from build123d import *

# Parameters (mm, degrees)
F0_W      = 78.632404
F0_H      = 78.044064
F1_DEPTH  = 19.05
F7_R      = 19.67966
F8_DEPTH  = 25.4
F9_R      = 25.337788
F10_DEPTH = 88.9
F11_W     = 78.605324
F11_H     = 78.906078
F12_DEPTH = 19.05
F13_R     = 19.066656
F14_DEPTH = 19.05
F6_R      = 6.832472
F15_DEPTH = 304.8
F4_R      = 6.169539
F16_DEPTH = 25.4
F3_R      = 6.600699
F17_DEPTH = 25.4
F5_R      = 6.490494
F18_DEPTH = 25.4
F19_R     = 6.482052
F19_R_2   = 6.426585
F19_R_3   = 6.219267
F19_R_4   = 6.38041
F20_DEPTH = 25.4


with BuildPart() as f1:
    # F0 (on Top) → F1 (new body)
    with BuildSketch(Plane.XY):
        with Locations((-12.092622, -33.094514)):
            Rectangle(F0_W, F0_H)
    extrude(amount=F1_DEPTH)

    # F7 (on face) → F8 (cut)
    with BuildSketch(Plane.XY.offset(19.05)):
        with Locations((-11.63225, -33.066146)):
            Circle(F7_R)
    extrude(amount=-F8_DEPTH, mode=Mode.SUBTRACT)

    # F9 (on face) → F10 (join)
    with BuildSketch(Plane.XY.offset(19.05)):
        with Locations((-11.359275, -33.27705)):
            Circle(F9_R)
    extrude(amount=F10_DEPTH)

    # F11 (on face) → F12 (join)
    with BuildSketch(Plane.XY.offset(107.95)):
        with Locations((-13.666842, -29.469063)):
            Rectangle(F11_W, F11_H)
    extrude(amount=F12_DEPTH)

    # F13 (on face) → F14 (cut)
    with BuildSketch(Plane.XY.offset(127)):
        with Locations((-13.757879, -30.534975)):
            Circle(F13_R)
    extrude(amount=-F14_DEPTH, mode=Mode.SUBTRACT)

    # F6 (on face) → F15 (cut)
    with BuildSketch(Plane.XY.offset(19.05)):
        with Locations((17.793169, -61.01913)):
            Circle(F6_R)
    extrude(amount=-F15_DEPTH, mode=Mode.SUBTRACT)

    # F4 (on face) → F16 (cut)
    with BuildSketch(Plane.XY.offset(19.05)):
        with Locations((17.894953, -2.897272)):
            Circle(F4_R)
    extrude(amount=-F16_DEPTH, mode=Mode.SUBTRACT)

    # F3 (on face) → F17 (cut)
    with BuildSketch(Plane.XY.offset(19.05)):
        with Locations((-42.325243, -4.469179)):
            Circle(F3_R)
    extrude(amount=-F17_DEPTH, mode=Mode.SUBTRACT)

    # F5 (on face) → F18 (cut)
    with BuildSketch(Plane.XY.offset(19.05)):
        with Locations((-40.706113, -62.110294)):
            Circle(F5_R)
    extrude(amount=-F18_DEPTH, mode=Mode.SUBTRACT)

    # F19 (on face) → F20 (cut)
    with BuildSketch(Plane.XY.offset(127)):
        with Locations((16.331086, 0)):
            Circle(F19_R)
        with Locations((16.997535, -59.755784)):
            Circle(F19_R_2)
        with Locations((-42.323295, -60.177404)):
            Circle(F19_R_3)
        with Locations((-42.10072, 0)):
            Circle(F19_R_4)
    extrude(amount=-F20_DEPTH, mode=Mode.SUBTRACT)


solid = f1.part
Build history of the part. All positions in model axes, mm. A direction names the side the tool comes from. Coordinates: 2 decimals unless noted, no trailing zeros. Order: outer loops, then holes, each group sorted by start corner. A loop starts at its lowest first (then second) coordinate and runs counter-clockwise, first axis right, second up. Notation, with made-up numbers: (-37, 78) - (9, 78) arc R29 cw to (9, 106) - close; hole circle Ø11 at (-16.75, 31). An arc over 180 degrees is marked (long way). Write item = value, one per line. Start each with the question number.
1) 3-axis set-ups, long thin cutter, end or side, ignore diameter. For faces 1 (the face through (25.636, -30, 117)), 2 (the face through (-47.26, -63.96, 117.61)), 3 (the face through (-51.409, -34, 9)), 4 (the face through (-32, -11, 107.95)): which of +Z, -Z, +X, -X, +Y, -Y reach the whole face in a straight line?
2) Saw through at C-C on z = 10.5. Write the cut outline in (x, y), then the cut area to 3 significant figures.
3) Saw through at D-D on y = -22. Write the cut outline in (x, z).
4) Wall check: line 1 along Z through (x, y) = (-28, -56); line 2 along X through (y, z) = (5, 108); line 3 along Z through (x, y) = (10.5, 6.5). Give the ranges that are in metal, low to high. Write a range as from..to.
5) Saw through at B-B on x = -17. Write the cut outline in (y, z), then the cut area to 3 significant figures.
6) Saw through at A-A on y = 0. Write the cut outline in (x, z).
7) Two-plate mould, pull along Y, no slides. Class faces 5 (the face through (-37.217, -56.637, 9.658)), 6 (the face through (-14, -68.922, 117)), 7 (the face through (-30, -24, 0)): pulls with the +Y half, pulls with the -Y half, needs draft (parallel to the pull), parting line crosses it, or undercut.
8) Flat gauge pins, fed straight in: pin 1 Ø20 at (x, y) = (-42.32, -60.18) entering from -Z; pin 2 Ø15 at (x, z) = (-26, 9) entering from +Y; pin 3 Ø1.5 at (x, z) = (-22.5, 89) entering from -Y; pin 4 Ø12 at (x, z) = (9.5, 111) entering from -Y. Where does each tip first touch, or does it go through?
From the geometry:
q1.face_1 = +Z, +X, +Y, -Y
q1.face_2 = +Z
q1.face_3 = -Z, -X, +Y, -Y
q1.face_4 = none
q2.outline = (-51.41, -72.12) - (27.22, -72.12) - (27.22, 5.93) - (-51.41, 5.93) - close; hole circle Ø13.2 at (-42.33, -4.47); hole circle Ø12.98 at (-40.71, -62.11); hole circle Ø39.36 at (-11.63, -33.07); hole circle Ø13.66 at (17.79, -61.02); hole circle Ø12.34 at (17.89, -2.9)
q2.area = 4,380 mm^2
q3.outline = (-52.97, 107.95) - (-34.05, 107.95) - (-34.05, 19.05) - (-51.41, 19.05) - (-51.41, 0) - (-27.91, 0) - (-27.91, 19.05) - (4.64, 19.05) - (4.64, 0) - (27.22, 0) - (27.22, 19.05) - (11.33, 19.05) - (11.33, 107.95) - (25.64, 107.95) - (25.64, 127) - (3.29, 127) - (3.29, 107.95) - (-30.81, 107.95) - (-30.81, 127) - (-52.97, 127) - close
q4.line_1 = 0..19.05, 107.95..127
q4.line_2 = -52.97..-46.06, -38.14..12.21, 20.46..25.64
q4.line_3 = 107.95..127
q5.outline = (-72.12, 0) - (-52, 0) - (-52, 19.05) - (-14.13, 19.05) - (-14.13, 0) - (5.93, 0) - (5.93, 19.05) - (-8.58, 19.05) - (-8.58, 107.95) - (9.98, 107.95) - (9.98, 127) - (-11.75, 127) - (-11.75, 107.95) - (-49.32, 107.95) - (-49.32, 127) - (-68.92, 127) - (-68.92, 107.95) - (-57.98, 107.95) - (-57.98, 19.05) - (-72.12, 19.05) - close
q5.area = 5,940 mm^2
q6.outline = (-52.97, 107.95) - (-48.48, 107.95) - (-48.48, 127) - (-52.97, 127) - close; (-51.41, 0) - (-47.18, 0) - (-47.18, 19.05) - (-51.41, 19.05) - close; (-37.47, 0) - (12.45, 0) - (12.45, 19.05) - (-37.47, 19.05) - close; (-35.72, 107.95) - (9.85, 107.95) - (9.85, 127) - (-35.72, 127) - close; (22.81, 107.95) - (25.64, 107.95) - (25.64, 127) - (22.81, 127) - close; (23.34, 0) - (27.22, 0) - (27.22, 19.05) - (23.34, 19.05) - close
q7.face_5 = undercut
q7.face_6 = pulls with the -Y half
q7.face_7 = needs draft
q8.pin_1 = 0
q8.pin_2 = 5.93
q8.pin_3 = -56.39
q8.pin_4 = -68.92
